from build123d import *

# Parameters (mm, degrees)
F0_W     = 47.0686554909
F0_H     = 47.0686554909
F1_DEPTH = 3


with BuildPart() as f1:
    # F0 (on Top) → F1 (new body)
    with BuildSketch(Plane.XY):
        with Locations((-15.658213757, 53.1422756612)):
            Rectangle(F0_W, F0_H)
        Polygon((7.8761139885, 29.6079479158), (-39.1925415024, 29.6079479158), (-39.1925415024, -17.4607075751), (7.8761139885, -17.4607075751), (54.9447694793, -17.4607075751), (54.9447694793, 29.6079479158), align=None)
        with Locations((-15.658213757, -40.9950353205)):
            Rectangle(F0_W, F0_H)
    extrude(amount=F1_DEPTH)


solid = f1.part
Input: part model. Units: mm. Frame: model coordinates. A direction names the side the tool comes from. Round coordinates to 2 decimals unless told otherwise and drop trailing zeros. Order: outer loops, then holes, each group sorted by start corner. A loop starts at its lowest first (then second) coordinate and runs counter-clockwise, first axis right, second up. Notation, with made-up numbers: (0, 79.25) - (23, 79.25) arc R5 cw to (23, 86.25) - close; hole circle Ø4 at (35.25, -30.75). An arc over 180 degrees is marked (long way). Use a Markdown table: item, result.
1. Section A-A on z = 0.7. Return the cut outline in (x, y).
Evaluation:
| item | result |
|---|---|
| outline | (-39.19, -64.53) - (7.88, -64.53) - (7.88, -17.46) - (54.94, -17.46) - (54.94, 29.61) - (7.88, 29.61) - (7.88, 76.68) - (-39.19, 76.68) - close |
2. Access query for faces 1 (the face through (-39.193, 7, 1)), 2 (the face through (32, 29.608, 1)), 3 (the face through (7.876, -41, 1)). Directions: +Z, -Z, +X, -X, +Y, -Y. A direction counts if a zero-diameter tool reaches every point of the face in a straight line with its end or side. Return the directions, or none.
Evaluation:
| item | result |
|---|---|
| face 1 | +Z, -Z, -X, +Y, -Y |
| face 2 | +Z, -Z, +X, +Y |
| face 3 | +Z, -Z, +X, -Y |
3. Material intervals for probe 1 along Y at (x, z) = (38.5, 0.4); probe 2 along X at (y, z) = (39, 0.85), sorted ascending.
Evaluation:
| item | result |
|---|---|
| probe 1 | -17.46 to 29.61 |
| probe 2 | -39.19 to 7.88 |
4. Section B-B on y = -41.5. Return the cut outline in (x, z), then the cut area to 3 significant figures.
Evaluation:
| item | result |
|---|---|
| outline | (-39.19, 0) - (7.88, 0) - (7.88, 3) - (-39.19, 3) - close |
| area | 141 mm^2 |
5. First-contact query: pin 1 (1.5 mm diameter, centred on x = 26, z = 1.5, fed in from -Y); pin 2 (3 mm diameter, centred on x = -8, y = 58.5, fed in from -Z); pin 3 (1.5 mm diameter, centred on y = 50, z = 1.5, fed in from +X). Flat tips, straight axial feed; report the tip coordinate or a pass-through.
Evaluation:
| item | result |
|---|---|
| pin 1 | y = -17.46 |
| pin 2 | z = 0 |
| pin 3 | x = 7.88 |
6. Section C-C on x = 23.5. Return the cut outline in (y, z).
Evaluation:
| item | result |
|---|---|
| outline | (-17.46, 0) - (29.61, 0) - (29.61, 3) - (-17.46, 3) - close |
